The listing builds one solid part. Answer for the finished solid, in the listing's coordinates (mm). Face numbers are marked on the shaded views. A direction names the side the tool comes from. Round coordinates to 2 decimals unless told otherwise and drop trailing zeros. Loops run counter-clockwise (first coordinate to the right, second up) from the corner with the lowest first, then second, coordinate; pieces in that order, holes last. Notation, with made-up numbers: (-37.5, -9) -> (-23.5, -9) arc R27 ccw to (-23.5, 14) -> close; hole circle Ø8 at (-38, 43). An arc over 180 degrees is marked (long way). Write each question's results on one line, items separated by ' | '. Start each with the question number.
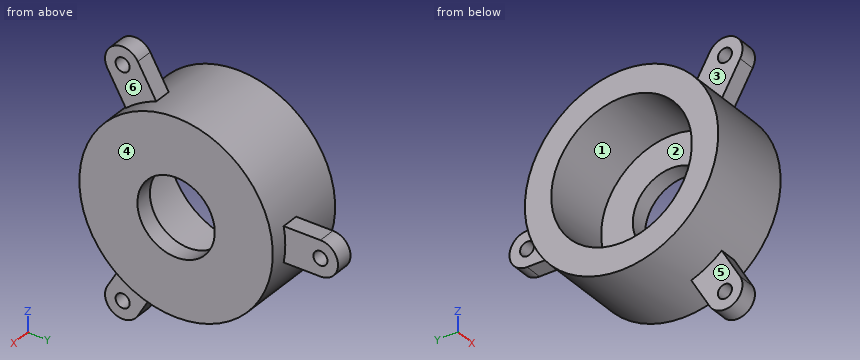
from build123d import *

# Parameters (mm, degrees)
BOSS_EXTRUDE1_START = -15
SKETCH4_R           = 4
BOSS_EXTRUDE1_DEPTH = 10
CIRPATTERN1_COUNT   = 3
SKETCH7_R           = 55
SKETCH7_R_2         = 22
CUT_EXTRUDE1_DEPTH  = 5


with BuildPart() as part:
    # Sketch3 → Revolve1 (revolve)
    with BuildSketch(Plane.XY, mode=Mode.PRIVATE) as revolve1_sk:
        Polygon((0, 40), (0, 55), (50, 55), (55, 55), (55, 52), (55, 22), (40, 22), (40, 40), align=None)
    revolve(revolve1_sk.sketch.rotate(Axis((-32.450781709, 0, 0), (1, 0, 0)), 90), axis=Axis((-32.450781709, 0, 0), (1, 0, 0)))

    # Sketch4 → Boss-Extrude1 (add)
    with BuildSketch(Plane(origin=(55, 0, 0), x_dir=(0, 0, -1), z_dir=(1, 0, 0)).offset(BOSS_EXTRUDE1_START)):
        with BuildLine():
            Line((10, 51.100551248), (10, 75))
            ThreePointArc((10, 75), (0, 85), (-10, 75))
            Line((-10, 75), (-10, 51.100551248))
            Line((-10, 51.100551248), (10, 51.100551248))
        make_face()
        with Locations((0, 75)):
            Circle(SKETCH4_R, mode=Mode.SUBTRACT)
    boss_extrude1 = extrude(amount=-BOSS_EXTRUDE1_DEPTH)

    # CirPattern1: Boss-Extrude1 ×3 about axis
    cirpattern1_axis = Axis((0, 0, 0), (1, 0, 0))
    for i in range(1, CIRPATTERN1_COUNT):
        add(boss_extrude1.rotate(cirpattern1_axis, i * 360 / CIRPATTERN1_COUNT))

    # Sketch7 → Cut-Extrude1 (cut)
    with BuildSketch(Plane(origin=(55, 0, 0), x_dir=(0, 0, -1), z_dir=(1, 0, 0))):
        with Locations(Location((0, 0, 0), (0, 0, 180))):
            Circle(SKETCH7_R)
        with Locations(Location((0, 0, 0), (0, 0, 180))):
            Circle(SKETCH7_R_2, mode=Mode.SUBTRACT)
    extrude(amount=-CUT_EXTRUDE1_DEPTH, mode=Mode.SUBTRACT)


solid = part.part
Item 1: Each of these flat-tipped pins is pushed along its axis until it touches: pin 1 Ø23.5 at (y, z) = (-31, -65.5) entering from -X; pin 2 Ø1.5 at (x, y) = (25, -12.5) entering from -Z; pin 3 Ø5 at (x, y) = (33, 63.5) entering from -Z; pin 4 Ø22 at (y, z) = (64.5, -3) entering from +X. Where does it stop, or does it pass through?
Item 2: The part is cut by section B-B, the plane y = 0. Give the vertices of the cut face in (x, z), plus the area to 3 significant figures.
Item 3: Determine the mould class of the marked faces 1, 2 and 3 for opening direction Y: +Y half, -Y half, draft (parallel to the pull), parting line (faces both ways), or undercut.
Item 4: For the marked faces 4, 5 and 6, determine the directions among +Z, -Z, +X, -X, +Y, -Y from which every point of the face is accessible in a straight line to the end or side of a thin tool.
Item 5: The part is cut by section C-C, the plane z = 18.5. Give the vertices of the cut face in (x, y).
Item 6: The part is cut by section A-A, the plane z = 0. Give the vertices of the cut face in (x, y).
Item 7: The part is cut by section D-D, the plane x = 25.5. Give the vertices of the cut face in (y, z), plus the area to 3 significant figures.
Item 8: Straight lines are drawn through the part: L1, parallel to Y at x = 31, z = 0; L2, parallel to Z at x = 35, y = -37; L3, parallel to Z at x = 33.5, y = 75. For each, find the intervals that lie inside material, in ascending order. Write a range as [from, to].
Report:
1) pin 1: stops at x = 30 | pin 2: stops at z = -53.73 | pin 3: stops at z = -10 | pin 4: stops at x = 50
2) outline: (0, -55) -> (50, -55) -> (50, -22) -> (40, -22) -> (40, -40) -> (0, -40) -> close; (0, 40) -> (40, 40) -> (40, 22) -> (50, 22) -> (50, 55) -> (0, 55) -> close | area: 1,860 mm2
3) face 1: undercut | face 2: undercut | face 3: draft
4) face 4: +Z, -Z, +X, +Y, -Y | face 5: -Z, -X, -Y | face 6: +Z, +X, -Y
5) outline: (0, -51.8) -> (50, -51.8) -> (50, -11.91) -> (40, -11.91) -> (40, -35.46) -> (0, -35.46) -> close; (0, 35.46) -> (40, 35.46) -> (40, 11.91) -> (50, 11.91) -> (50, 51.8) -> (0, 51.8) -> close
6) outline: (0, -55) -> (50, -55) -> (50, -22) -> (40, -22) -> (40, -40) -> (0, -40) -> close; (0, 40) -> (40, 40) -> (40, 22) -> (50, 22) -> (50, 55) -> (40, 55) -> (40, 71) -> (30, 71) -> (30, 55) -> (0, 55) -> close; (30, 79) -> (40, 79) -> (40, 85) -> (30, 85) -> close
7) outline: circle Ø110 at (0, 0); hole circle Ø80 at (0, 0) | area: 4,480 mm2
8) L1: y = [-55, -40], [40, 71], [79, 85] | L2: z = [-74.94, -68.92], [-60.98, -44.09], [-40.69, -15.2], [15.2, 40.69], [44.09, 60.98], [68.92, 74.94] | L3: z = [-10, -4], [4, 10]
